Geometry check sheet. Reference: drawing and pictorial views, mm from the part's lowest x, y, z. A direction names the side the tool comes from. Round coordinates to 2 decimals unless told otherwise and drop trailing zeros. Write each loop counter-clockwise with the first axis right and the second up, starting at its lowest first coordinate (ties: lowest second). Pieces come first, ordered by that corner, then holes. Notation, with made-up numbers: (41.5, 46) -> (95.5, 46) arc R12 ccw to (95.5, 54) -> close; hole circle Ø11 at (49, 6). An arc over 180 degrees is marked (long way). Answer as a JSON object with one key per item and string values. Group by question number.
(1) Draft check along X on the marked faces 1, 2 and 3. Enter one of: released by +X, released by -X, zero draft, split by the parting line, or undercut.
(2) Sectioned sample at A-A on y = 52.5. Record the cut outline in (x, z), and give its area (3 significant figures).
(3) Scan lines: L1, parallel to X at y = 4.5, z = 13.15; L2, parallel to Y at x = 95.25, z = 13.15; L3, parallel to X at y = 9, z = 9.5. Record each from-to range of solid material in increasing order. Write a range as from..to.
(4) Sectioned sample at C-C on x = 19.35. Record the cut outline in (y, z).
(5) Sectioned sample at D-D on x = 60. Record the cut outline in (y, z).
(6) Gauge pin test, flat ends, axial feed: pin 1 Ø11 at (y, z) = (22.5, 13.15) entering from -X; pin 2 Ø6 at (x, z) = (73.5, 22) entering from +Y. Record the tip position at first contact, or that the pin passes through.
(7) Set-up check for the marked faces 4 and 5: record each of +Z, -Z, +X, -X, +Y, -Y from which the full face is reachable in a straight line by a thin tool's end or side.
(8) Sectioned sample at B-B on z = 29.15. Record the cut outline in (x, y).
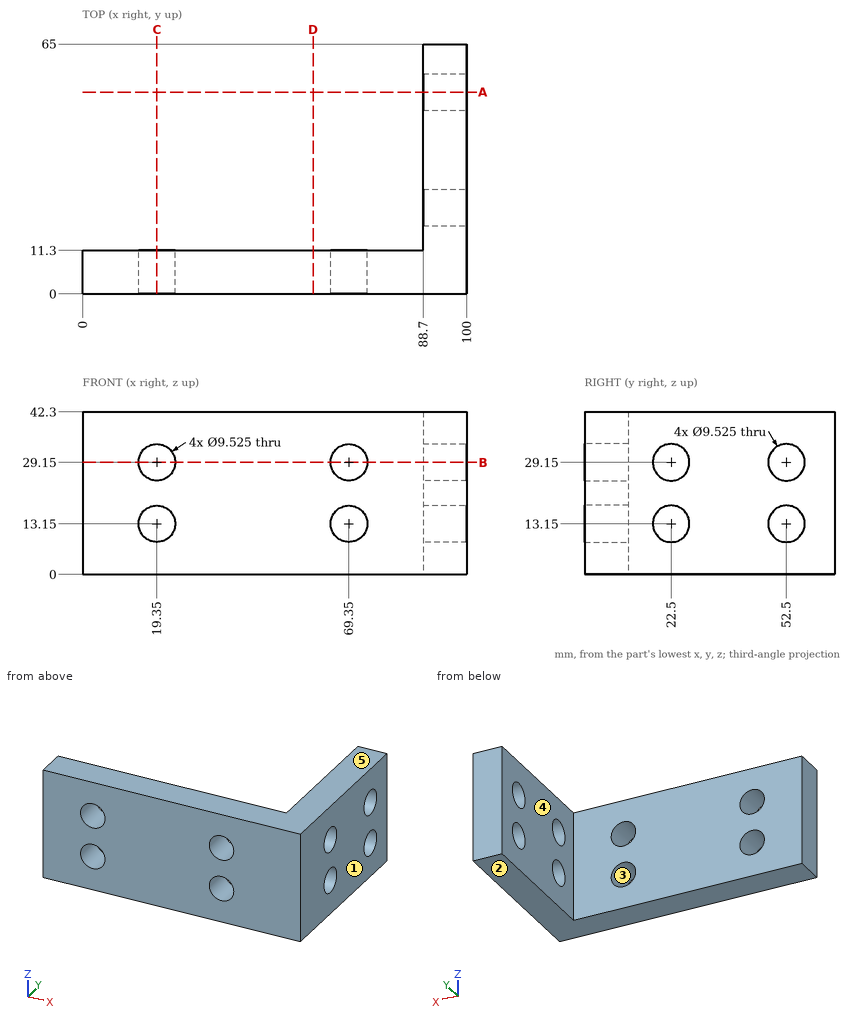
Computed values:
{
 "1": {"face 1": "released by +X", "face 2": "zero draft", "face 3": "undercut"},
 "2": {"outline": "(88.7, 0) -> (100, 0) -> (100, 8.39) -> (88.7, 8.39) -> close; (88.7, 17.91) -> (100, 17.91) -> (100, 24.39) -> (88.7, 24.39) -> close; (88.7, 33.91) -> (100, 33.91) -> (100, 42.3) -> (88.7, 42.3) -> close", "area": "263 mm2"},
 "3": {"L1": "0..14.59, 24.11..64.59, 74.11..100", "L2": "0..17.74, 27.26..47.74, 57.26..65", "L3": "0..16.29, 22.41..66.29, 72.41..100"},
 "4": {"outline": "(0, 0) -> (11.3, 0) -> (11.3, 8.39) -> (0, 8.39) -> close; (0, 17.91) -> (11.3, 17.91) -> (11.3, 24.39) -> (0, 24.39) -> close; (0, 33.91) -> (11.3, 33.91) -> (11.3, 42.3) -> (0, 42.3) -> close"},
 "5": {"outline": "(0, 0) -> (11.3, 0) -> (11.3, 42.3) -> (0, 42.3) -> close"},
 "6": {"pin 1": "x = 88.7", "pin 2": "y = 11.3"},
 "7": {"face 4": "+Z, -Z, -X, +Y", "face 5": "+Z, +X, -X, +Y, -Y"},
 "8": {"outline": "(0, 0) -> (14.59, 0) -> (14.59, 11.3) -> (0, 11.3) -> close; (24.11, 0) -> (64.59, 0) -> (64.59, 11.3) -> (24.11, 11.3) -> close; (74.11, 0) -> (100, 0) -> (100, 17.74) -> (88.7, 17.74) -> (88.7, 11.3) -> (74.11, 11.3) -> close; (88.7, 27.26) -> (100, 27.26) -> (100, 47.74) -> (88.7, 47.74) -> close; (88.7, 57.26) -> (100, 57.26) -> (100, 65) -> (88.7, 65) -> close"}
}
